```python
from build123d import *

# Parameters (mm, degrees)
PAD041_DEPTH    = 15
SKETCH095_R     = 2.5
POCKET045_DEPTH = 5
SKETCH096_R     = 2.4
PAD042_DEPTH    = 5


with BuildPart() as part:
    # Sketch094 → Pad041 (new body)
    with BuildSketch(Plane.XY):
        Polygon((30.122286, 194.043034), (13.580843, 194.042587), (4.144071, 199.977952), (-15.017249, 203.244653), (-16.854137, 203.244653), (-18.898529, 205.918312), (4.128235, 205.918312), (30.122286, 205.918312), (30.122286, 199.855942), align=None)
    extrude(amount=PAD041_DEPTH)

    # Sketch095 (on Face3 of Pad041) → Pocket045 (cut)
    with BuildSketch(Plane(origin=(33.2471900087, 195.0163320297, 0), x_dir=(0.9857768846, -0.1680593161, 0), z_dir=(-0.1680593161, -0.9857768846, 0))):
        with Locations((-43.193441, 7.824432)):
            Circle(SKETCH095_R)
    extrude(amount=-POCKET045_DEPTH, mode=Mode.SUBTRACT)

    # Sketch096 (on Face1 of Pocket045) → Pad042 (join)
    with BuildSketch(Plane(origin=(-0.0052436098, 194.0422198627, 0), x_dir=(0.9999999996, 2.7023e-05, 0), z_dir=(2.7023e-05, -0.9999999996, 0))):
        with Locations((17.901974, 7.158432)):
            Circle(SKETCH096_R)
        with Locations((26.5802, 7.158432)):
            Circle(SKETCH096_R)
    extrude(amount=PAD042_DEPTH)


with BuildPart() as part_1:
    # Body012 placement: moved
    add(part.part.moved(Location((0, 0, -65))))


solid = part_1.part
```
Geometry: final body of the model. Coordinates: model frame, mm. A direction names the side the tool comes from. Give positions to 0.01 mm unless a question says otherwise; leave off trailing zeros. Order: outer loops, then holes, each group sorted by start corner. A loop starts at its lowest first (then second) coordinate and runs counter-clockwise, first axis right, second up. Notation, with made-up numbers: (-7, 20.25) -> (0, 20.25) arc R23 cw to (0, 35.25) -> close; hole circle Ø8 at (-25, 88). An arc over 180 degrees is marked (long way). Write each question's results on one line, items separated by ' | '. Start each with the question number.
1) Line query: line 1 (Y direction, x = 22.5, z = -53); line 2 (X direction, y = 192.25, z = -55.75); line 3 (Z direction, x = -9.5, y = 203.75). Output: solid intervals per line, ascending. Write a range as from..to.
2) Section C-C (y = 196.25). Return loops of the section in (x, z), then the cut area to 3 significant figures.
3) Section A-A (z = -64). Return loops of the section in (x, y).
4) Section B-B (z = -56.5). Return loops of the section in (x, y).
5) Section D-D (x = 12). Return loops of the section in (y, z), then the cut area to 3 significant figures.
6) Set-up query: faces 4 (the flat face through (30.122, 200, -58)), 5 (the flat face through (-16, 203.245, -58)). Return all of +Z, -Z, +X, -X, +Y, -Y with unobstructed straight access to the full face (end or side cutting, diameter ignored); none if empty.
7) First-contact query: pin 1 (5 mm diameter, centred on x = 23, z = -62.5, fed in from -Y); pin 2 (8 mm diameter, centred on y = 203, z = -58.5, fed in from -X); pin 3 (3 mm diameter, centred on x = -10.5, z = -56, fed in from -Y). Flat tips, straight axial feed; report the tip coordinate or a pass-through.
8) Draft query along X for faces 1 (the cylindrical face through (27.68, 191.58, -59.97)), 2 (the flat face through (11, 201, -65)), 3 (the flat face through (-5.3, 201.59, -57.6)). Return one class per face: pulls with the +X half, pulls with the -X half, needs draft (parallel to the pull), parting line crosses it, or undercut.
Calculated:
1) line 1: 194.04..205.92 | line 2: 16.72..19.07, 25.4..27.75 | line 3: -65..-59.64, -54.71..-50
2) outline: (10.07, -65) -> (30.12, -65) -> (30.12, -50) -> (10.07, -50) -> close | area: 301 mm2
3) outline: (-18.9, 205.92) -> (-16.85, 203.24) -> (-15.02, 203.24) -> (4.14, 199.98) -> (13.58, 194.04) -> (30.12, 194.04) -> (30.12, 205.92) -> close
4) outline: (-18.9, 205.92) -> (-16.85, 203.24) -> (-15.02, 203.24) -> (-11.7, 202.68) -> (-11.15, 205.92) -> close; (-6.96, 201.87) -> (4.14, 199.98) -> (13.58, 194.04) -> (15.91, 194.04) -> (15.91, 189.04) -> (19.89, 189.04) -> (19.89, 194.04) -> (24.58, 194.04) -> (24.59, 189.04) -> (28.57, 189.04) -> (28.56, 194.04) -> (30.12, 194.04) -> (30.12, 205.92) -> (-6.27, 205.92) -> close
5) outline: (195.04, -65) -> (205.92, -65) -> (205.92, -50) -> (195.04, -50) -> close | area: 163 mm2
6) face 4: +Z, -Z, +X, +Y, -Y | face 5: +Z, -Z, -X, -Y
7) pin 1: y = 194.04 | pin 2: x = -18.9 | pin 3: y = 202.34
8) face 1: undercut | face 2: needs draft | face 3: pulls with the -X half
